Answer from the drawing. Dimensions are ordinates in mm from the lowest x, y and z of the part. A direction names the side the tool comes from. Round coordinates to 2 decimals unless told otherwise and drop trailing zeros. Order: outer loops, then holes, each group sorted by start corner. A loop starts at its lowest first (then second) coordinate and runs counter-clockwise, first axis right, second up. Notation, with made-up numbers: M 11,43.25 L 32,43.25 A25 cw 32,58.25 Z; hole C 10.5,57.25 d7. An arc over 180 degrees is marked long. Answer as a JSON object with one key per item and string values. Group by question number.
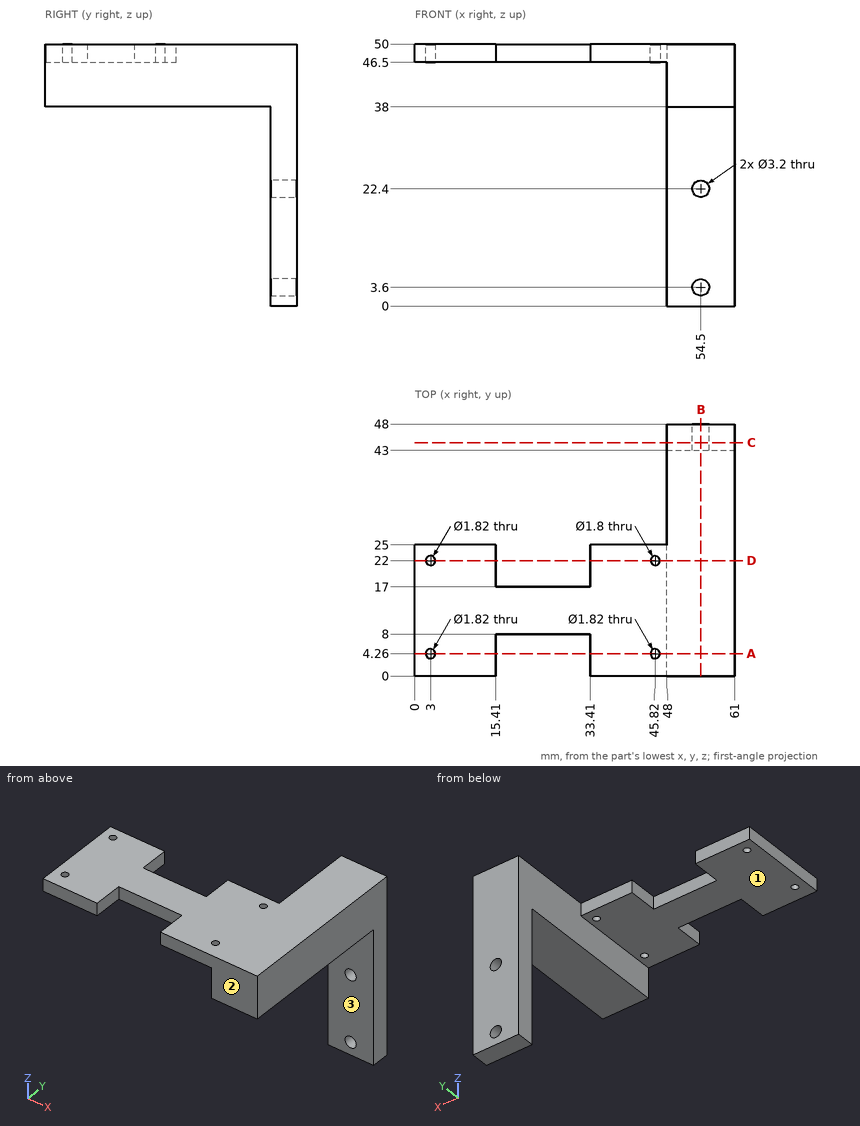
Item 1: Find section D-D (y = 22). Give the vertices of the cut face in (x, z), and give its area (3 significant figures).
Item 2: A tool of negligible diameter and unlimited length cuts with its end or side. For the marked faces 1, 2 and 3, from which of +Z, -Z, +X, -X, +Y, -Y can it reach the whole face along a straight path? Write none if from no direction.
Item 3: Each of these flat-tipped pins is pushed along its axis until it touches: pin 1 (1.8 mm diameter, centred on x = 24.5, z = 48.5, fed in from -Y); pin 2 (7.5 mm diameter, centred on x = 13.5, y = 17, fed in from -Z); pin 3 (2.5 mm diameter, centred on x = 54.5, z = 3.6, fed in from -Y); pin 4 (1 mm diameter, centred on x = 10, z = 48, fed in from +Y). Where does it stop, or does it pass through?
Item 4: Find section B-B (x = 54.5). Give the vertices of the cut face in (y, z), and give its area (3 significant figures).
Item 5: Find section C-C (y = 44.5). Give the vertices of the cut face in (x, z), and give its area (3 significant figures).
Item 6: Find section A-A (y = 4.26). Give the vertices of the cut face in (x, z), and give its area (3 significant figures).
Item 7: Consider L1, parallel to X at y = 22, z = 48; L2, parallel to Y at x = 45.82, z = 49; L3, parallel to X at y = 44, z = 31.5. Determine where each line is inside the solid, lowest interval first.
Responses:
{
 "1": {"outline": "M 0,46.5 L 2.09,46.5 L 2.09,50 L 0,50 Z; M 3.91,46.5 L 15.41,46.5 L 15.41,50 L 3.91,50 Z; M 33.41,46.5 L 44.92,46.5 L 44.92,50 L 33.41,50 Z; M 46.72,46.5 L 48,46.5 L 48,38 L 61,38 L 61,50 L 46.72,50 Z", "area": "248 mm^2"},
 "2": {"face 1": "-Z, -X, +Y, -Y", "face 2": "+Z, -Z, +X, -X, -Y", "face 3": "-Z, +X, -X, -Y"},
 "3": {"pin 1": "stops at y = 8", "pin 2": "stops at z = 46.5", "pin 3": "passes through", "pin 4": "stops at y = 25"},
 "4": {"outline": "M 0,38 L 43,38 L 43,24 L 48,24 L 48,50 L 0,50 Z; M 43,0 L 48,0 L 48,2 L 43,2 Z; M 43,5.2 L 48,5.2 L 48,20.8 L 43,20.8 Z", "area": "734 mm^2"},
 "5": {"outline": "M 48,0 L 61,0 L 61,50 L 48,50 Z; hole C 54.5,3.6 d3.2; hole C 54.5,22.4 d3.2", "area": "634 mm^2"},
 "6": {"outline": "M 0,46.5 L 2.09,46.5 L 2.09,50 L 0,50 Z; M 3.91,46.5 L 15.41,46.5 L 15.41,50 L 3.91,50 Z; M 33.41,46.5 L 44.91,46.5 L 44.91,50 L 33.41,50 Z; M 46.73,46.5 L 48,46.5 L 48,38 L 61,38 L 61,50 L 46.73,50 Z", "area": "248 mm^2"},
 "7": {"L1": "x = 0 to 2.09, 3.91 to 15.41, 33.41 to 44.92, 46.72 to 61", "L2": "y = 0 to 3.35, 5.17 to 21.1, 22.9 to 25", "L3": "x = 48 to 61"}
}
